The model under review builds one solid part; all positions refer to its coordinate system, in mm. A direction names the side the tool comes from. Round coordinates to 2 decimals unless told otherwise and drop trailing zeros. Write each loop counter-clockwise with the first axis right and the second up, starting at its lowest first coordinate (ties: lowest second). Pieces come first, ordered by that corner, then holes. Notation, with made-up numbers: (52, 0) - (102, 0) arc R26 ccw to (102, 27) - close; hole circle Ø3 at (5, 23.25). An arc over 180 degrees is marked (long way). Use one line per item in the form item = value.
from build123d import *

# Parameters (mm, degrees)
SKETCH_1_W          = 89
SKETCH_1_H          = 10
EXTRUDE_1_DEPTH     = 30
SKETCH_2_R          = 21.15
CUT_EXTRUDE_1_DEPTH = 20
SKETCH_3_R          = 1.7
CUT_EXTRUDE_2_DEPTH = 60
SKETCH_4_R          = 3.7
CUT_EXTRUDE_3_DEPTH = 10
FILLET_START        = -5
FILLET_1_DEPTH      = 10


with BuildPart() as part:
    # 草图1 → 凸台-拉伸1 (new body)
    with BuildSketch(Plane(origin=(0, 0, 0), x_dir=(1, 0, 0), z_dir=(0, 1, 0))):
        Rectangle(SKETCH_1_W, SKETCH_1_H)
    extrude(amount=EXTRUDE_1_DEPTH)

    # 草图2 → 切除-拉伸1 (cut)
    with BuildSketch(Plane.XY.offset(5)):
        Circle(SKETCH_2_R)
    extrude(amount=-CUT_EXTRUDE_1_DEPTH, mode=Mode.SUBTRACT)

    # 草图3 → 切除-拉伸2 (cut)
    with BuildSketch(Plane.XZ):
        with Locations(Location((-30, 0, 0), (0, 0, 270))):
            Circle(SKETCH_3_R)
        with Locations(Location((30, 0, 0), (0, 0, 270))):
            Circle(SKETCH_3_R)
    extrude(amount=-CUT_EXTRUDE_2_DEPTH, mode=Mode.SUBTRACT)

    # 草图4 → 切除-拉伸3 (cut)
    with BuildSketch(Plane(origin=(0, 30, 0), x_dir=(1, 0, 0), z_dir=(0, 1, 0))):
        with Locations(Location((-30, 0, 0), (0, 0, 270))):
            Circle(SKETCH_4_R)
        with Locations(Location((30, 0, 0), (0, 0, 270))):
            Circle(SKETCH_4_R)
    extrude(amount=-CUT_EXTRUDE_3_DEPTH, mode=Mode.SUBTRACT)

    # 圆角1: read off the stored shape, not the designer's step
    # 圆角1 outline → 圆角1 (cut)
    with BuildSketch(Plane.XY.offset(FILLET_START)):
        with BuildLine():
            ThreePointArc((-44.5, 0), (-35.713203436, 21.213203436), (-14.5, 30))
            Line((-14.5, 30), (-44.5, 30))
            Line((-44.5, 30), (-44.5, 0))
        make_face()
        with BuildLine():
            ThreePointArc((14.5, 30), (35.713203436, 21.213203436), (44.5, 0))
            Line((44.5, 0), (44.5, 30))
            Line((44.5, 30), (14.5, 30))
        make_face()
    extrude(amount=FILLET_1_DEPTH, mode=Mode.SUBTRACT)


solid = part.part
(1) Add section D-D on y = 19. Write out the cut boundary in (x, z).
Geometry results:
outline = (-37.72, -5) - (-9.29, -5) - (-9.29, 5) - (-37.72, 5) - close; (9.29, -5) - (37.72, -5) - (37.72, 5) - (9.29, 5) - close; hole circle Ø3.4 at (-30, 0); hole circle Ø3.4 at (30, 0)
(2) Add section A-A on y = 14. Write out the cut boundary in (x, z), then the cut area to 3 significant figures.
Geometry results:
outline = (-41.03, -5) - (-15.85, -5) - (-15.85, 5) - (-41.03, 5) - close; (15.85, -5) - (41.03, -5) - (41.03, 5) - (15.85, 5) - close; hole circle Ø3.4 at (-30, 0); hole circle Ø3.4 at (30, 0)
area = 485 mm2
(3) Add section B-B on z = 0. Write out the cut boundary in (x, y).
Geometry results:
outline = (-44.5, 0) - (-31.7, 0) - (-31.7, 20) - (-33.7, 20) - (-33.7, 23.05) arc R30 ccw to start; (-28.3, 0) - (-21.15, 0) arc R21.15 cw to (21.15, 0) - (28.3, 0) - (28.3, 20) - (26.3, 20) - (26.3, 27.58) arc R30 ccw to (14.5, 30) - (-14.5, 30) arc R30 ccw to (-26.3, 27.58) - (-26.3, 20) - (-28.3, 20) - close; (31.7, 0) - (44.5, 0) arc R30 ccw to (33.7, 23.05) - (33.7, 20) - (31.7, 20) - close
(4) Machinability: for faces 5 (the flat face through (-32, 20, 1)), 6 (the flat face through (-0.6, 21.5, 5)), which of the approach directions +Z, -Z, +X, -X, +Y, -Y give a long, thin tool a straight path to every point of the face, cutting with its end or side? Answer none if there is none.
Geometry results:
face_5 = +Y
face_6 = +Z, +X, -X, +Y, -Y
(5) Add section C-C on x = 30. Write out the cut boundary in (y, z).
Geometry results:
outline = (0, -5) - (25.69, -5) - (25.69, -3.7) - (20, -3.7) - (20, -1.7) - (0, -1.7) - close; (0, 1.7) - (20, 1.7) - (20, 3.7) - (25.69, 3.7) - (25.69, 5) - (0, 5) - close
(6) To check wall thickness, follow L1, parallel to Z at x = -30, y = 24.75; L2, parallel to X at y = 15.25, z = 0; L3, parallel to X at y = 7.5, z = 0.5. State the ranges of each line that lie inside material, in increasing order.
Geometry results:
L1 = -5 to -3.7, 3.7 to 5
L2 = -40.33 to -31.7, -28.3 to -14.65, 14.65 to 28.3, 31.7 to 40.33
L3 = -43.55 to -31.62, -28.38 to -19.78, 19.78 to 28.38, 31.62 to 43.55
(7) Insertion check: P1, Ø1.5, axis at y = 14.5, z = -1, coming from the +X side; P2, Ø6, axis at x = 31, z = 3, coming from the +Y side; P3, Ø4.5, axis at x = -30, z = 0, coming from the +Y side. Each pin has a flat end and moves straight along its axis. Give the tip position at first contact, or say it passes through.
Geometry results:
P1 = 41.16
P2 = 26.79
P3 = 20
(8) The part is to be moulded in two halves that separate along X. For faces 1 (the flat face through (33, 0, 0)), 2 (the cylindrical face through (-35.945, 20.979, -0.07)), 3 (the cylindrical face through (35.479, 21.445, -0.07)), 4 (the cylindrical face through (28.34, 9.86, 0.37)), say which applies: +X half, -X half, draft (parallel to the pull), parting line (faces both ways), or undercut.
Geometry results:
face_1 = draft
face_2 = -X half
face_3 = +X half
face_4 = undercut
